Geometry: final body of the model. Coordinates: model frame, mm. Coordinates: 2 decimals unless noted, no trailing zeros. Loops run counter-clockwise (first coordinate to the right, second up) from the corner with the lowest first, then second, coordinate; pieces in that order, holes last. Notation, with made-up numbers: (-25.5, 20.5) - (6.5, 20.5) arc R19 ccw to (6.5, 50.5) - close; hole circle Ø8 at (57, 79). An arc over 180 degrees is marked (long way). Put each result on its own line as item: value. Start each with the question number.
1) Section B-B on z = -11.5. Output: boundary loops of the cut face in (x, y), and give its area (3 significant figures).
2) Material intervals for line 1 along Z through (x, y) = (3, -1.2); line 2 along X through (y, z) = (-0.75, 14.5); line 3 along X through (y, z) = (-0.25, -8), sorted ascending. Write a range as from..to.
3) Section C-C on z = 18. Output: boundary loops of the cut face in (x, y), and give its area (3 significant figures).
4) Section A-A on x = -3. Output: boundary loops of the cut face in (y, z), and give its area (3 significant figures).
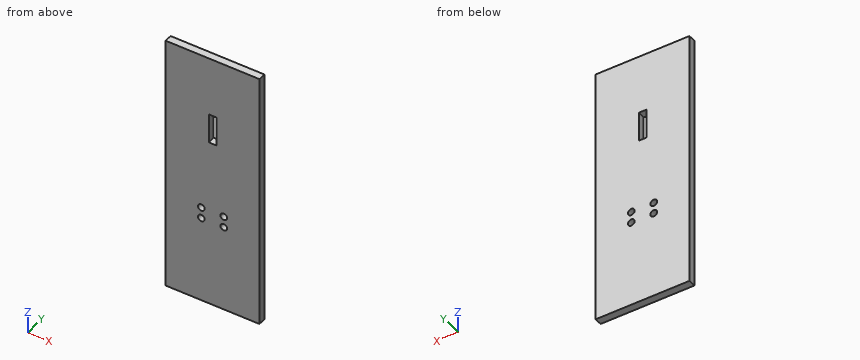
```python
from build123d import *

# Parameters (mm, degrees)
F0_W     = 25
F0_H     = 70
F0_R     = 0.9
F0_W_2   = 2
F0_H_2   = 8
F1_DEPTH = 2


with BuildPart() as f1:
    # F0 (on Front) → F1 (new body)
    with BuildSketch(Plane.XZ):
        Rectangle(F0_W, F0_H)
        with Locations((-3, -11.5)):
            Circle(F0_R, mode=Mode.SUBTRACT)
        with Locations((-3, -8.5)):
            Circle(F0_R, mode=Mode.SUBTRACT)
        with Locations((3, -11.5)):
            Circle(F0_R, mode=Mode.SUBTRACT)
        with Locations((3, -8.5)):
            Circle(F0_R, mode=Mode.SUBTRACT)
        with Locations((0, 15)):
            Rectangle(F0_W_2, F0_H_2, mode=Mode.SUBTRACT)
    extrude(amount=F1_DEPTH)


solid = f1.part
```
Answer block:
1. outline: (-12.5, -2) - (-3.9, -2) - (-3.9, 0) - (-12.5, 0) - close; (-2.1, -2) - (2.1, -2) - (2.1, 0) - (-2.1, 0) - close; (3.9, -2) - (12.5, -2) - (12.5, 0) - (3.9, 0) - close
1. area: 42.8 mm²
2. line 1: z = -35..-12.4, -10.6..-9.4, -7.6..35
2. line 2: x = -12.5..-1, 1..12.5
2. line 3: x = -12.5..-3.75, -2.25..2.25, 3.75..12.5
3. outline: (-12.5, -2) - (-1, -2) - (-1, 0) - (-12.5, 0) - close; (1, -2) - (12.5, -2) - (12.5, 0) - (1, 0) - close
3. area: 46.0 mm²
4. outline: (-2, -35) - (0, -35) - (0, -12.4) - (-2, -12.4) - close; (-2, -10.6) - (0, -10.6) - (0, -9.4) - (-2, -9.4) - close; (-2, -7.6) - (0, -7.6) - (0, 35) - (-2, 35) - close
4. area: 133 mm²
